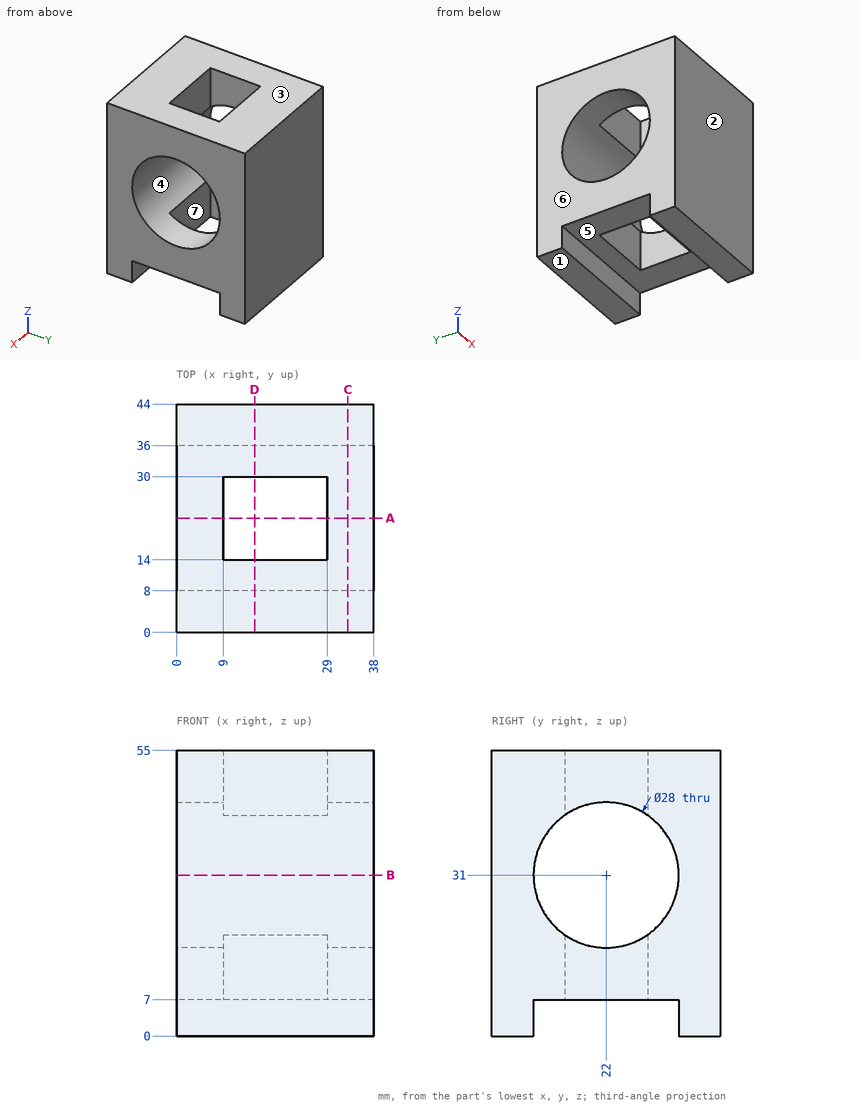
Here's the drawing with two shaded views (mm, measured from the low corner). I have some questions. A direction names the side the tool comes from. Round coordinates to 2 decimals unless told otherwise and drop trailing zeros. Order: outer loops, then holes, each group sorted by start corner. A loop starts at its lowest first (then second) coordinate and runs counter-clockwise, first axis right, second up. Notation, with made-up numbers: (-0.75, 8) -> (36.25, 8) arc R20 ccw to (36.25, 43) -> close; hole circle Ø1 at (-35, 76.25). An arc over 180 degrees is marked (long way). Write each question's results on one line, items separated by ' | '. Start each with the question number.
Item 1: If we section it at B-B, the plane z = 31: Write out the boundary of the cut face in (x, y).
Item 2: If we section it at D-D, the plane x = 15: Write out the boundary of the cut face in (y, z), then the cut area to 3 significant figures.
Item 3: Which directions (+Z, -Z, +X, -X, +Y, -Y) give clear straight access to the entire face, cutting with the end or side of a thin tool? Please do the marked faces 5, 6 and 7.
Item 4: Thinking about a two-plate mould opening in Z: for the marked faces 1, 2, 3 and 4, which applies, +Z half, -Z half, draft (parallel to the pull), parting line (faces both ways), or undercut?
Item 5: If we section it at A-A, the plane y = 22: Write out the boundary of the cut face in (x, z), then the cut area to 3 significant figures.
Item 6: Will this pin go through, and if not, where does the flat tip stop? pin 1 (6 mm diameter, centred on x = 30, y = 29, fed in from -Z).
Item 7: Please list where these lines run through material, in increasing order: L1, parallel to Z at x = 6.5, y = 30; L2, parallel to X at y = 29.5, z = 46; L3, parallel to Y at x = 22.5, z = 47.
Item 8: If we section it at C-C, the plane x = 33: Write out the boundary of the cut face in (y, z).
Results:
1) outline: (0, 0) -> (38, 0) -> (38, 8) -> (0, 8) -> close; (0, 36) -> (38, 36) -> (38, 44) -> (0, 44) -> close
2) outline: (0, 0) -> (8, 0) -> (8, 7) -> (14, 7) -> (14, 19.51) arc R14 cw to (14, 42.49) -> (14, 55) -> (0, 55) -> close; (30, 7) -> (36, 7) -> (36, 0) -> (44, 0) -> (44, 55) -> (30, 55) -> (30, 42.49) arc R14 cw to (30, 19.51) -> close | area: 1,260 mm2
3) face 5: -Z, +X, -X | face 6: +Z, -Z, -X, +Y, -Y | face 7: +Z, -Z
4) face 1: -Z half | face 2: draft | face 3: +Z half | face 4: undercut
5) outline: (0, 7) -> (9, 7) -> (9, 17) -> (0, 17) -> close; (0, 45) -> (9, 45) -> (9, 55) -> (0, 55) -> close; (29, 7) -> (38, 7) -> (38, 17) -> (29, 17) -> close; (29, 45) -> (38, 45) -> (38, 55) -> (29, 55) -> close | area: 360 mm2
6) pin 1: stops at z = 7
7) L1: z = 7 to 19.51, 42.49 to 55 | L2: x = 0 to 9, 29 to 38 | L3: y = 0 to 14, 30 to 44
8) outline: (0, 0) -> (8, 0) -> (8, 7) -> (36, 7) -> (36, 0) -> (44, 0) -> (44, 55) -> (0, 55) -> close; hole circle Ø28 at (22, 31)
